Geometry: final body of the model. Coordinates: model frame, mm. Coordinates: 2 decimals unless noted, no trailing zeros. Loops run counter-clockwise (first coordinate to the right, second up) from the corner with the lowest first, then second, coordinate; pieces in that order, holes last. Notation, with made-up numbers: (39, 35) - (56, 35) arc R26 ccw to (56, 51) - close; hole circle Ø4 at (12.25, -27). An arc over 180 degrees is marked (long way). Answer in a Markdown table with one row per item.
from build123d import *

# Parameters (mm, degrees)
F0_R     = 19.05
F1_DEPTH = 10.16
F2_T     = -4.318
F3_R     = 5.08


# Not quite as in the source:
# - a fillet or chamfer that OpenCascade refuses, or shapes differently, is made with other operations: its cross-section is extruded or revolved along the edge and cut away or added


with BuildPart() as f1:
    # F0 (on Front) → F1 (new body)
    with BuildSketch(Plane.XZ):
        Circle(F0_R)
    extrude(amount=F1_DEPTH)

    # F2
    f2_openings = [f1.faces().sort_by_distance(p)[0] for p in [
        (0, -10.16, 0),
    ]]
    offset(amount=F2_T, openings=f2_openings)

    # F3
    f3_edges = [f1.edges().sort_by_distance(p)[0] for p in [
        (-14.732, -4.318, 0),
    ]]
    fillet(f3_edges, radius=F3_R)

    # F4: fillet of radius 5.08 on 1 edges, made by hand

    # F4_s1 → F4_t2 (revolve, cut)
    with BuildSketch(Plane.XY):
        with BuildLine():
            ThreePointArc((14.2503822155, -7.239), (16.1249178862, -9.3680135261), (18.848764431, -10.16))
            Line((18.848764431, -10.16), (18.848764431, -10.668))
            Line((18.848764431, -10.668), (14.732, -10.668))
            Line((14.732, -10.668), (14.224, -10.16))
            ThreePointArc((14.224, -10.16), (14.224, -9.398), (13.790543994, -7.4549))
            Line((13.790543994, -7.4549), (14.2503822155, -7.239))
        make_face()
    revolve(axis=Axis((0, -10.16, 0), (0, -1, 0)), mode=Mode.SUBTRACT)

    # F5: fillet of radius 5.08 on 1 edges, made by hand

    # F5_s1 → F5_t2 (revolve, cut)
    with BuildSketch(Plane.XY):
        with BuildLine():
            ThreePointArc((18.848764431, -10.16), (18.9994394971, -9.4592919765), (19.05, -8.7443525768))
            Line((19.05, -8.7443525768), (19.05, -10.16))
            Line((19.05, -10.16), (18.848764431, -10.16))
        make_face()
    revolve(axis=Axis((0, -10.16, 0), (0, -1, 0)), mode=Mode.SUBTRACT)


solid = f1.part
(1) Cut plane A-A on z = 0. Output: boundary loops of the cut face in (x, y), then the cut area to 3 significant figures.
Verdict:
| item | result |
|---|---|
| outline | (-19.05, -8.74) arc R5.08 ccw to (-18.85, -10.16) arc R5.08 ccw to (-14.25, -7.24) arc R5.08 cw to (-9.65, -4.32) - (9.65, -4.32) arc R5.08 cw to (14.25, -7.24) arc R5.08 ccw to (18.85, -10.16) arc R5.08 ccw to (19.05, -8.74) - (19.05, 0) - (-19.05, 0) - close |
| area | 220 mm² |
(2) First-contact query: pin 1 Ø6 at (x, y) = (-6.5, -8) entering from +Z; pin 2 Ø1 at (x, z) = (-13.5, 3.5) entering from -Y; pin 3 Ø6 at (x, z) = (-14, 1) entering from -Y. Flat tips, straight axial feed; report the tip coordinate or a pass-through.
Verdict:
| item | result |
|---|---|
| pin 1 | stops at z = 18.73 |
| pin 2 | stops at y = -7.61 |
| pin 3 | stops at y = -9.83 |
(3) Cut plane D-D on y = -3.5. Output: boundary loops of the cut face in (x, z), then the cut area to 3 significant figures.
Verdict:
| item | result |
|---|---|
| outline | circle Ø38.1 at (0, 0) |
| area | 1,140 mm² |
(4) Cut plane B-B on x = 0. Output: boundary loops of the cut face in (y, z), then the cut area to 3 significant figures.
Verdict:
| item | result |
|---|---|
| outline | (-10.16, -18.85) arc R5.08 ccw to (-8.74, -19.05) - (0, -19.05) - (0, 19.05) - (-8.74, 19.05) arc R5.08 ccw to (-10.16, 18.85) arc R5.08 ccw to (-7.24, 14.25) arc R5.08 cw to (-4.32, 9.65) - (-4.32, -9.65) arc R5.08 cw to (-7.24, -14.25) arc R5.08 ccw to start |
| area | 220 mm² |
(5) Pull-direction query (Z, two-part tool) for faces 1 (the face through (-15.12, -4.31, -11.59)), 2 (the face through (0, 0, 0)), 3 (the face through (0, -4.318, 0)); classes: pulls with the +Z half, pulls with the -Z half, needs draft (parallel to the pull), parting line crosses it, or undercut.
Verdict:
| item | result |
|---|---|
| face 1 | parting line crosses it |
| face 2 | needs draft |
| face 3 | undercut |
(6) Ray query, probe 1 along Y at (x, z) = (5.5, -4); probe 2 along Y at (x, z) = (-5, -11.5); probe 3 along X at (y, z) = (-2.25, 17.5). Return the intervals inside material, ascending.
Verdict:
| item | result |
|---|---|
| probe 1 | y = -4.32 to 0 |
| probe 2 | y = -5.22 to 0 |
| probe 3 | x = -7.53 to 7.53 |
(7) Cut plane C-C on y = -5.5. Output: boundary loops of the cut face in (x, z), then the cut area to 3 significant figures.
Verdict:
| item | result |
|---|---|
| outline | circle Ø38.1 at (0, 0); hole circle Ø25.82 at (0, 0) |
| area | 617 mm² |
